```python
from build123d import *

# Parameters (mm, degrees)
BOSS_EXTRUDE1_DEPTH         = 5
MIRROR1_DEPTH               = 5
SCALE1_SCALE                = 0.6
SCALE2_SCALE_X              = 0.5
SCALE2_SCALE_Y              = 1
SCALE2_SCALE_Z              = 1
SKETCH2_W                   = 9
SKETCH2_H                   = 6
CUT_EXTRUDE1_DEPTH          = 98.801494894
BODY_MOVE_COPY1_START       = 1
BODY_MOVE_COPY1_DEPTH       = 3
BODY_MOVE_COPY1_2_OUTLINE_W = 9
BODY_MOVE_COPY1_2_OUTLINE_H = 6
BODY_MOVE_COPY1_2_DEPTH     = 3


# Read off the part's stored shape, not the designer's step: Mirror1, Body-Move/Copy1
with BuildPart() as part:
    # Sketch1 → Boss-Extrude1 (new body)
    with BuildSketch(Plane(origin=(0, 0, 0), x_dir=(1, 0, 0), z_dir=(0, 1, 0))):
        with BuildLine():
            Line((0, 0), (0, 11.771243445))
            Line((0, 11.771243445), (20, 11.771243445))
            ThreePointArc((20, 11.771243445), (26.771243445, 6.771243445), (35, 5))
            Line((35, 5), (75, 5))
            Line((75, 5), (75, 0))
            Line((75, 0), (0, 0))
        make_face()
    extrude(amount=BOSS_EXTRUDE1_DEPTH)

    # Mirror1 outline → Mirror1 (add)
    with BuildSketch(Plane(origin=(0, 0, 0), x_dir=(1, 0, 0), z_dir=(0, 1, 0))):
        with BuildLine():
            Line((115, 5), (75, 5))
            Line((75, 5), (75, 0))
            Line((75, 0), (0, 0))
            Line((0, 0), (0, -11.771243445))
            Line((0, -11.771243445), (20, -11.771243445))
            ThreePointArc((20, -11.771243445), (26.771243445, -6.771243445), (35, -5))
            Line((35, -5), (115, -5))
            ThreePointArc((115, -5), (123.228756555, -6.771243445), (130, -11.771243445))
            Line((130, -11.771243445), (150, -11.771243445))
            Line((150, -11.771243445), (150, 11.771243445))
            Line((150, 11.771243445), (130, 11.771243445))
            ThreePointArc((130, 11.771243445), (123.228756555, 6.771243445), (115, 5))
        make_face()
    extrude(amount=MIRROR1_DEPTH)


with BuildPart() as part_1:
    # Scale1: scaled about (75, 2.5, 0)
    add(part.part.scale(SCALE1_SCALE).moved(Location((30, 1, 0))))


with BuildPart() as part_2:
    # Scale2: scaled about (75, 2.5, 0)
    add(part_1.part.scale((SCALE2_SCALE_X, SCALE2_SCALE_Y, SCALE2_SCALE_Z), about=(75, 2.5, 0)))

    # Sketch2 → Cut-Extrude1 (cut, through all)
    with BuildSketch(Plane(origin=(0, 4, 0), x_dir=(1, 0, 0), z_dir=(0, 1, 0))):
        with Locations((70.5, 0)):
            Rectangle(SKETCH2_W, SKETCH2_H)
    extrude(amount=-CUT_EXTRUDE1_DEPTH, mode=Mode.SUBTRACT)


with BuildPart() as cut_extrude1_piece_1:
    # of the separate pieces the step leaves, piece 1, a body of its own (cut_extrude1_pieces)
    add(part_2.part.solids().sort_by_distance((75, 1, 3))[0])

    # Body-Move/Copy1 outline → Body-Move/Copy1 (cut)
    with BuildSketch(Plane(origin=(0, 0, 0), x_dir=(1, 0, 0), z_dir=(0, 1, 0)).offset(BODY_MOVE_COPY1_START)):
        with BuildLine():
            add(Edge.make_bspline(
                [(91.5, 7.062746067), (90.655623636, 5.147880462), (89.601040636, 3.949624901), (88.5, 3.381049961)],
                knots=[0.344491118, 0.344491118, 0.344491118, 0.344491118, 0.443649167, 0.443649167, 0.443649167, 0.443649167], degree=3, weights=[0.571428571, 0.621399531, 0.697590007, 0.8]))
            Line((88.5, 3.381049961), (88.5, -3.381049961))
            add(Edge.make_bspline(
                [(88.5, -3.381049961), (89.601040636, -3.949624901), (90.655623636, -5.147880462), (91.5, -7.062746067)],
                knots=[0.056350833, 0.056350833, 0.056350833, 0.056350833, 0.155508882, 0.155508882, 0.155508882, 0.155508882], degree=3, weights=[0.8, 0.697590007, 0.621399531, 0.571428571]))
            Line((91.5, -7.062746067), (97.5, -7.062746067))
            Line((97.5, -7.062746067), (97.5, 7.062746067))
            Line((97.5, 7.062746067), (91.5, 7.062746067))
        make_face()
    extrude(amount=BODY_MOVE_COPY1_DEPTH, mode=Mode.SUBTRACT)

    # Body-Move_Copy1 2 outline → Body-Move_Copy1 2 (add)
    with BuildSketch(Plane(origin=(0, 0, 0), x_dir=(1, 0, 0), z_dir=(0, 1, 0)).offset(BODY_MOVE_COPY1_START)):
        with BuildLine():
            Line((88.5, 7.062746067), (82.5, 7.062746067))
            add(Edge.make_bspline(
                [(82.5, 7.062746067), (81.233643288, 4.190918983), (79.569499126, 3), (78, 3)],
                knots=[0.344491118, 0.344491118, 0.344491118, 0.344491118, 0.5, 0.5, 0.5, 0.5], degree=3, weights=[0.571428571, 0.649797681, 0.792654824, 1]))
            Line((78, 3), (87, 3))
            add(Edge.make_bspline(
                [(88.5, 3.381049961), (87.991386346, 3.118403), (87.487429398, 3), (87, 3)],
                knots=[0.443649167, 0.443649167, 0.443649167, 0.443649167, 0.5, 0.5, 0.5, 0.5], degree=3, weights=[0.8, 0.85819889, 0.924865556, 1]))
            Line((88.5, 3.381049961), (88.5, 7.062746067))
        make_face()
        with Locations((70.5, 0)):
            Rectangle(BODY_MOVE_COPY1_2_OUTLINE_W, BODY_MOVE_COPY1_2_OUTLINE_H)
        with BuildLine():
            Line((88.5, -7.062746067), (88.5, -3.381049961))
            add(Edge.make_bspline(
                [(87, -3), (87.487429398, -3), (87.991386346, -3.118403), (88.5, -3.381049961)],
                knots=[0, 0, 0, 0, 0.056350833, 0.056350833, 0.056350833, 0.056350833], degree=3, weights=[1, 0.924865556, 0.85819889, 0.8]))
            Line((87, -3), (78, -3))
            add(Edge.make_bspline(
                [(78, -3), (79.569499126, -3), (81.233643288, -4.190918983), (82.5, -7.062746067)],
                knots=[0, 0, 0, 0, 0.155508882, 0.155508882, 0.155508882, 0.155508882], degree=3, weights=[1, 0.792654824, 0.649797681, 0.571428571]))
            Line((82.5, -7.062746067), (88.5, -7.062746067))
        make_face()
    extrude(amount=BODY_MOVE_COPY1_2_DEPTH)


with BuildPart() as cut_extrude1_piece_2:
    # of the separate pieces the step leaves, piece 2, a body of its own (cut_extrude1_pieces)
    add(part_2.part.solids().sort_by_distance((52.5, 1, -7.062746067))[0])


with BuildPart() as cut_extrude1_piece_1_1:
    add(cut_extrude1_piece_1.part)

    # Combine1: union Cut-Extrude1 piece 2
    add(cut_extrude1_piece_2.part)


solid = cut_extrude1_piece_1_1.part
```
For this review, take the finished solid that the model builds, in its own axes (mm). A direction names the side the tool comes from. Round coordinates to 2 decimals unless told otherwise and drop trailing zeros. Write each loop counter-clockwise with the first axis right and the second up, starting at its lowest first coordinate (ties: lowest second). Pieces come first, ordered by that corner, then holes. Notation, with made-up numbers: (76.25, 40.25) -> (117.25, 40.25) arc R36 ccw to (117.25, 76.25) -> close; hole circle Ø8 at (-37.5, 67.5). An arc over 180 degrees is marked (long way). One line per question, with ' | ' between items. Start each with the question number.
(1) Mouldability with a two-part tool opening along X and no side actions: class faces 3 (the face through (86, 2, -7.063)), 4 (the face through (88.5, 2, 0)), 5 (the face through (70, 2, 3)) as released by +X, released by -X, zero draft, split by the parting line, or undercut.
(2) Add section A-A, the plane x = 68. Write out the cut boundary in (y, z), plus the area to 3 significant figures.
(3) Tool access review of faces 1 (the face through (71, 2, -3)), 2 (the face through (70, 4, 0)): name each direction out of +Z, -Z, +X, -X, +Y, -Y from which nothing blocks a thin tool from reaching the whole face with its end or side.
(4) For line 1 along Z through (x, y) = (70, 1.4); line 2 along X through (y, z) = (1.9, 4.5); line 3 along X through (y, z) = (2.45, 5), list the stretches that pass through material, from the lowest coordinate up. Write a range as from..to.
Answer list:
1) face 3: zero draft | face 4: released by +X | face 5: undercut
2) outline: (1, -3) -> (4, -3) -> (4, 3) -> (1, 3) -> close | area: 18.0 mm²
3) face 1: -Z, +Y, -Y | face 2: +Z, -Z, +X, -X, +Y
4) line 1: -3..3 | line 2: 52.5..60.1, 80.9..88.5 | line 3: 52.5..59.68, 81.32..88.5
